Design review of the part built by this model. Coordinates are the model's own, in mm. Face numbers are marked on the shaded views. A direction names the side the tool comes from. Give positions to 0.01 mm unless a question says otherwise; leave off trailing zeros. Write each loop counter-clockwise with the first axis right and the second up, starting at its lowest first coordinate (ties: lowest second). Pieces come first, ordered by that corner, then holes. Notation, with made-up numbers: M 76.5,-11.5 L 81.5,-11.5 A19 cw 81.5,-5.5 Z; hole C -26,-15.5 d8. An arc over 180 degrees is marked long. Answer in a Markdown table with one row per item.
Autodesk Inventor part; units mm, degrees
ref_plane "XZ Plane" through (0, 0, 0) normal (0, 1, 0) x (-1, 0, 0)
ref_plane "XY Plane" through (0, 0, 0) normal (0, 0, 1) x (1, 0, 0)
sketch "Sketch1" plane through (0, 0, 0) normal (0, 1, 0) x (-1, 0, 0)
  circle A0 centre (0, 0) radius 8
  dimension "d0" = 16
extrude "Extrusion1" add sketch "Sketch1" along normal blind 2
sketch "Sketch2" plane through (0, 2, 0) normal (0, 1, 0) x (1, 0, 0)
  circle A0 centre (0, 0) radius 6.5
  dimension "d3" = 13
extrude "Extrusion2" add sketch "Sketch2" along normal blind 1.5
sketch "Sketch3" plane through (0, 3.5, 0) normal (0, 1, 0) x (1, 0, 0)
  circle A0 centre (0, 0) radius 8
  dimension "d6" = 16
extrude "Extrusion3" add sketch "Sketch3" along normal blind 2
sketch "Sketch4" plane through (0, 5.5, 0) normal (0, 1, 0) x (1, 0, 0)
  circle A0 centre (2.5, 0) radius 5.5
  circle A1 centre (0, 0) radius 8
  dimension "d9" = 11
extrude "Extrusion4" add sketch "Sketch4" along normal blind 4 contours A0
ref_plane "Work Plane1" through (8, 5.5, 0) normal (1, 0, 0) x (0, 1, 0)
sketch "Sketch5" plane through (8, 5.5, 0) normal (1, 0, 0) x (0, 1, 0)
  line L0 (4, -5.5) -> (4, 5.5)
  point P0 (-5.5, 0)
  point P1 (2, 0)
  dimension "d12" = 2
hole "Hole1" at (8, 7.5, 0) direction (-1, 0, 0) diameter 2.5 depth 2.15 tip angle 118
thread "Thread1"
sketch "Sketch6" plane through (2.5, 9.5, 0) normal (0, 1, 0) x (1, 0, 0)
  point P0 (-2.5, 0)
  point P1 (0, 0)
hole "Hole2" at (2.5, 9.5, 0) direction (0, -1, 0) diameter 7 end through all
properties material "Steel, Mild"
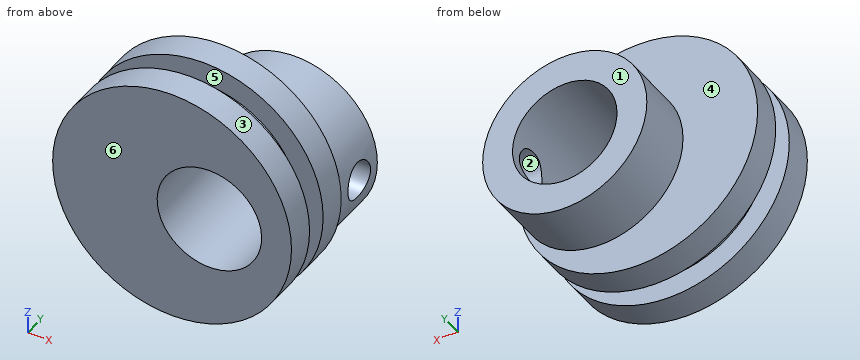
1) To check wall thickness, follow probe 1 along Y at (x, z) = (7.25, 0); probe 2 along Y at (x, z) = (5.75, 3.5); probe 3 along Y at (x, z) = (-6.25, -3.25). State the ranges of each line that lie inside material, in increasing order. Write a range as [from, to].
Geometry says:
| item | result |
|---|---|
| probe 1 | [0, 2], [3.5, 6.25], [8.75, 9.5] |
| probe 2 | [0, 2], [3.5, 9.5] |
| probe 3 | [0, 2], [3.5, 5.5] |
2) For the marked faces 4, 5 and 6, list the 3-axis set-ups (+Z, -Z, +X, -X, +Y, -Y) from which the entire face can be reached by the end or side of a thin tool; tool diameter is ignored.
Geometry says:
| item | result |
|---|---|
| face 4 | +Y |
| face 5 | none |
| face 6 | +Z, -Z, +X, -X, -Y |
3) Add section D-D (z = 4.5). Write out the cut boundary in (x, y), and give its area (3 significant figures).
Geometry says:
| item | result |
|---|---|
| outline | M -6.61,0 L 6.61,0 L 6.61,2 L 4.69,2 L 4.69,3.5 L 6.61,3.5 L 6.61,5.5 L 5.66,5.5 L 5.66,9.5 L -0.66,9.5 L -0.66,5.5 L -6.61,5.5 L -6.61,3.5 L -4.69,3.5 L -4.69,2 L -6.61,2 Z |
| area | 92.3 mm^2 |
4) Add section B-B (x = 0.75). Write out the cut boundary in (y, z).
Geometry says:
| item | result |
|---|---|
| outline | M 0,-7.96 L 2,-7.96 L 2,-6.46 L 3.5,-6.46 L 3.5,-7.96 L 5.5,-7.96 L 5.5,-5.21 L 9.5,-5.21 L 9.5,-3.03 L 0,-3.03 Z; M 0,3.03 L 9.5,3.03 L 9.5,5.21 L 5.5,5.21 L 5.5,7.96 L 3.5,7.96 L 3.5,6.46 L 2,6.46 L 2,7.96 L 0,7.96 Z |
5) The part is to be moulded in two halves that separate along Y. For the marked faces 1, 2 and 3, say which applies: released by +Y, released by -Y, zero draft, split by the parting line, or undercut.
Geometry says:
| item | result |
|---|---|
| face 1 | released by +Y |
| face 2 | undercut |
| face 3 | zero draft |
6) Insertion check: P1, Ø1, axis at y = 4, z = -5, coming from the +X side; P2, Ø2, axis at y = 4.5, z = -2, coming from the -X side; P3, Ø3, axis at y = 7.5, z = 0, coming from the -X side. Each pin has a flat end and moves straight along its axis. Give the tip position at first contact, or say it passes through.
Geometry says:
| item | result |
|---|---|
| P1 | x = 6.61 |
| P2 | x = -7.94 |
| P3 | x = -3 |
7) Add section C-C (y = 3.25). Write out the cut boundary in (x, z).
Geometry says:
| item | result |
|---|---|
| outline | C 0,0 d13; hole C 2.5,0 d7 |
8) Add section A-A (x = 7). Write out the cut boundary in (y, z).
Geometry says:
| item | result |
|---|---|
| outline | M 0,-3.87 L 2,-3.87 L 2,3.87 L 0,3.87 Z; M 3.5,-3.87 L 5.5,-3.87 L 5.5,-3.16 L 9.5,-3.16 L 9.5,3.16 L 5.5,3.16 L 5.5,3.87 L 3.5,3.87 Z; hole C 7.5,0 d2.5 |
